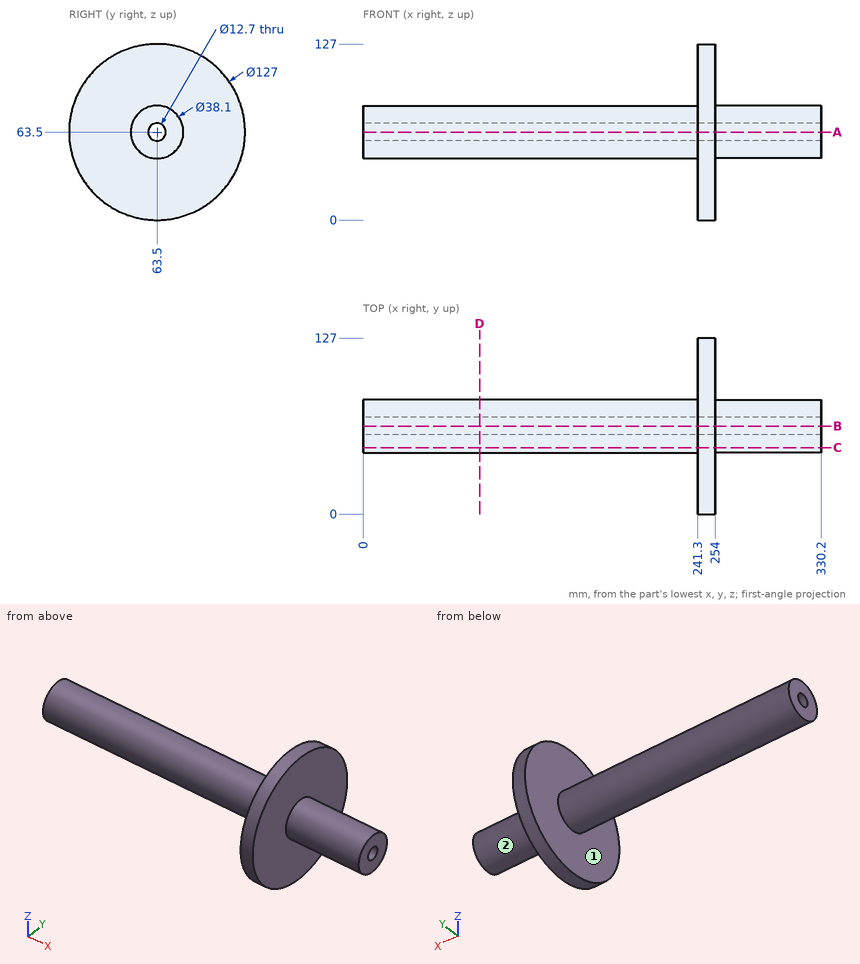
Check sheet for the drawn part. Datum: minimum x, y, z corner. Units: mm. A direction names the side the tool comes from. Round coordinates to 2 decimals unless told otherwise and drop trailing zeros. Order: outer loops, then holes, each group sorted by start corner. A loop starts at its lowest first (then second) coordinate and runs counter-clockwise, first axis right, second up.
1. Section check C-C on y = 48. Record the cut outline in (x, z).
Final values:
outline: (0, 52.43) - (241.3, 52.43) - (241.3, 1.92) - (254, 1.92) - (254, 52.43) - (330.2, 52.43) - (330.2, 74.57) - (254, 74.57) - (254, 125.08) - (241.3, 125.08) - (241.3, 74.57) - (0, 74.57) - close
2. Section check A-A on z = 63.5. Record the cut outline in (x, y).
Final values:
outline: (0, 44.45) - (241.3, 44.45) - (241.3, 0) - (254, 0) - (254, 44.45) - (330.2, 44.45) - (330.2, 57.15) - (0, 57.15) - close; (0, 69.85) - (330.2, 69.85) - (330.2, 82.55) - (254, 82.55) - (254, 127) - (241.3, 127) - (241.3, 82.55) - (0, 82.55) - close
3. Thickness scan on L1, parallel to Z at x = 236, y = 63.5; L2, parallel to Z at x = 252, y = 63; L3, parallel to Y at x = 216, z = 63. Record the ranges inside material, lowest first.
Final values:
L1: z = 44.45 to 57.15, 69.85 to 82.55
L2: z = 0 to 57.17, 69.83 to 127
L3: y = 44.46 to 57.17, 69.83 to 82.54
4. Access from +Z, -Z, +X, -X, +Y, -Y to the whole of each face (thin tool, end or side, straight path). Record for the marked faces 1 and 2.
Final values:
face 1: -X
face 2: +X
5. Section check D-D on x = 84. Record the cut outline in (y, z).
Final values:
outline: circle Ø38.1 at (63.5, 63.5); hole circle Ø12.7 at (63.5, 63.5)
6. Go/stop test with flat-tipped pins: P1, Ø10, axis at x = 203, y = 34.5, coming from the -Z side; P2, Ø5, axis at y = 17, z = 76, coming from the -X side; P3, Ø1.5, axis at x = 130, z = 53, coming from the -Y side; P4, Ø12, axis at x = 148.5, z = 83, coming from the -Y side. Record where each tip stops, or that it passes through.
Final values:
P1: passes through
P2: stops at x = 241.3
P3: stops at y = 47.13
P4: stops at y = 50.06
